Geometry: final body of the model. Coordinates: model frame, mm. Face numbers are marked on the shaded views. A direction names the side the tool comes from. Round coordinates to 2 decimals unless told otherwise and drop trailing zeros. Loops run counter-clockwise (first coordinate to the right, second up) from the corner with the lowest first, then second, coordinate; pieces in that order, holes last. Notation, with made-up numbers: M -5.75,59 L 7.25,59 A7 ccw 7.25,72 Z; hole C 9,-27.75 d10. An arc over 180 degrees is marked long. Return JSON: item names as keys, results as strings.
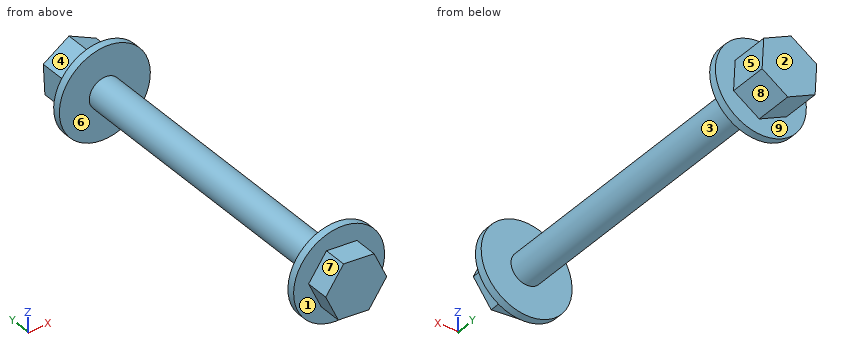
from build123d import *

# Parameters (mm, degrees)
SKETCH1_R           = 3.2639
BOSS_EXTRUDE1_DEPTH = 63.5
SKETCH2_R           = 9.525
BOSS_EXTRUDE2_DEPTH = 1.5875
BOSS_EXTRUDE3_START = 1.5875
SKETCH3_R           = 9.525
BOSS_EXTRUDE3_DEPTH = 1.5875
BOSS_EXTRUDE4_DEPTH = 4.7625
BOSS_EXTRUDE5_DEPTH = 7.9375


with BuildPart() as part:
    # Sketch1 → Boss-Extrude1 (new body)
    with BuildSketch(Plane(origin=(0, 0, 0), x_dir=(1, 0, 0), z_dir=(0, 1, 0))):
        with Locations(Location((0, 0, 0), (0, 0, 270))):
            Circle(SKETCH1_R)
    extrude(amount=BOSS_EXTRUDE1_DEPTH)

    # Sketch2 → Boss-Extrude2 (add)
    with BuildSketch(Plane(origin=(0, 63.5, 0), x_dir=(1, 0, 0), z_dir=(0, 1, 0))):
        with Locations(Location((0, 0, 0), (0, 0, 270))):
            Circle(SKETCH2_R)
    extrude(amount=BOSS_EXTRUDE2_DEPTH)

    # Sketch3 → Boss-Extrude3 (add)
    with BuildSketch(Plane.XZ.offset(BOSS_EXTRUDE3_START)):
        with Locations(Location((0, 0, 0), (0, 0, 90))):
            Circle(SKETCH3_R)
    extrude(amount=-BOSS_EXTRUDE3_DEPTH)

    # Sketch4 → Boss-Extrude4 (add)
    with BuildSketch(Plane.XZ.offset(1.5875)):
        Polygon((3.739867225, 5.213055267), (-2.64470468, 5.845347658), (-6.384571906, 0.63229239), (-3.739867225, -5.213055267), (2.64470468, -5.845347658), (6.384571906, -0.63229239), align=None)
    extrude(amount=BOSS_EXTRUDE4_DEPTH)

    # Sketch5 → Boss-Extrude5 (add)
    with BuildSketch(Plane(origin=(0, 65.0875, 0), x_dir=(1, 0, 0), z_dir=(0, 1, 0))):
        Polygon((5.379355204, -3.496439571), (5.717683093, 2.910438477), (0.33832789, 6.406878048), (-5.379355204, 3.496439571), (-5.717683093, -2.910438477), (-0.33832789, -6.406878048), align=None)
    extrude(amount=BOSS_EXTRUDE5_DEPTH)


solid = part.part
Q1. Reachability of the marked faces 5, 6, 7, 8 and 9 from +Z, -Z, +X, -X, +Y, -Y: full face, straight path, thin tool, end or side. Return the list, or none.
Determined:
{"face 5": "+Z, +X, +Y", "face 6": "none", "face 7": "+Z, -X, -Y", "face 8": "-Z, +X, +Y", "face 9": "+Y"}
Q2. Section query A-A (z = 8.5). Output: boundary loops of the cut face in (x, y), plus the area to 3 significant figures.
Determined:
{"outline": "M -4.3,-1.59 L 4.3,-1.59 L 4.3,0 L -4.3,0 Z; M -4.3,63.5 L 4.3,63.5 L 4.3,65.09 L -4.3,65.09 Z", "area": "27.3 mm^2"}
Q3. Section query B-B (y = 58). Output: boundary loops of the cut face in (x, z).
Determined:
{"outline": "C 0,0 d6.53"}
Q4. Pull-direction query (Y, two-part tool) for the marked faces 1, 2, 3 and 4; classes: pulls with the +Y half, pulls with the -Y half, needs draft (parallel to the pull), parting line crosses it, or undercut.
Determined:
{"face 1": "pulls with the -Y half", "face 2": "pulls with the +Y half", "face 3": "undercut", "face 4": "needs draft"}
Q5. Pin query (flat end, axial travel): pin 1 (3 mm diameter, centred on x = -6, y = 44.5, fed in from +Z); pin 2 (4 mm diameter, centred on y = 20, z = -0.5, fed in from +X); pin 3 (10 mm diameter, centred on y = 51.5, z = -4.5, fed in from -X); pin 4 (5 mm diameter, centred on x = 3.5, y = 16, fed in from +Z). Return the tip coordinate at first contact, or that it passes through.
Determined:
{"pin 1": "passes through", "pin 2": "stops at x = 3.26", "pin 3": "stops at x = -3.26", "pin 4": "stops at z = 3.11"}
Q6. Material intervals for L1, parallel to Y at x = 4.5, z = -2.25 (3 decimals); L2, parallel to Y at x = -6.5, z = -1; L3, parallel to X at y = 48.5, z = 0, sorted ascending.
Determined:
{"L1": "y = -6.35 to 0, 63.5 to 73.025", "L2": "y = -1.59 to 0, 63.5 to 65.09", "L3": "x = -3.26 to 3.26"}
